CAD build for the part. Positions are in the model's coordinates, mm. A direction names the side the tool comes from. Coordinates: 2 decimals unless noted, no trailing zeros. Order: outer loops, then holes, each group sorted by start corner. A loop starts at its lowest first (then second) coordinate and runs counter-clockwise, first axis right, second up. Notation, with made-up numbers: M 24,58 L 82,58 A22 ccw 82,96 Z; hole C -5.5,59 d8. An arc over 180 degrees is marked long. One line per item, written item: value.
from build123d import *

# Parameters (mm, degrees)
F0_W     = 87.5153616071
F0_H     = 111.0227331519
F1_DEPTH = 60.452
F2_W     = 61.5649223328
F2_H     = 93.4719592333
F3_DEPTH = 25.4
F4_DEPTH = 25.4
F5_DEPTH = 25.4
F6_R     = 10.9826729048
F7_DEPTH = 111.0237331519
F8_W     = 35.9690990299
F8_H     = 23.0667970557
F9_DEPTH = 87.5163616071


with BuildPart() as f1:
    # F0 (on Top) → F1 (new body)
    with BuildSketch(Plane.XY):
        Rectangle(F0_W, F0_H)
    extrude(amount=F1_DEPTH)

    # F2 (on face) → F3 (cut)
    with BuildSketch(Plane.XY.offset(60.452)):
        Rectangle(F2_W, F2_H)
    extrude(amount=-F3_DEPTH, mode=Mode.SUBTRACT)

    # F4 (cut): a face of the model
    f4_faces = [f1.faces().sort_by_distance(p)[0] for p in [
        (0, 0, 35.052),
    ]]
    extrude(f4_faces, amount=-F4_DEPTH, mode=Mode.SUBTRACT)

    # F5 (cut): a face of the model
    f5_faces = [f1.faces().sort_by_distance(p)[0] for p in [
        (0, 0, 9.652),
    ]]
    extrude(f5_faces, amount=-F5_DEPTH, mode=Mode.SUBTRACT)

    # F6 (on face) → F7 (cut, through all)
    with BuildSketch(Plane(origin=(0, 55.511366576, 0), x_dir=(-1, 0, 0), z_dir=(0, 1, 0))):
        with Locations((0, 30.2436631173)):
            Circle(F6_R)
    extrude(amount=-F7_DEPTH, mode=Mode.SUBTRACT)

    # F8 (on face) → F9 (cut, through all)
    with BuildSketch(Plane(origin=(-43.7576808035, 0, 0), x_dir=(0, -1, 0), z_dir=(-1, 0, 0))):
        with Locations((0.5664424971, 48.9186014721)):
            Rectangle(F8_W, F8_H)
    extrude(amount=-F9_DEPTH, mode=Mode.SUBTRACT)


solid = f1.part
Q1. Which spindle directions (+Z, -Z, +X, -X, +Y, -Y) get a long thin tool onto all of the face, cutting with end or side? Do faces 1 (the face through (30.782, -1, 31)), 2 (the face through (37, 17.418, 49)), 3 (the face through (-10, 55.511, 37)). Say none if no direction does.
Recorded:
face 1: +Z, -Z
face 2: +Z, +X, -X
face 3: +Z, -Z, +X, -X, +Y
Q2. Mould opens along Y. For faces 4 (the face through (1.43, 51.185, 41.133)), 5 (the face through (-10, -55.511, 37)), 6 (the face through (-37, 0, 37.385)) say: released by +Y, released by -Y, zero draft, split by the parting line, or undercut.
Recorded:
face 4: zero draft
face 5: released by -Y
face 6: undercut
Q3. Slice it at B-B (y = -45). List the corners of the cut face in (x, z).
Recorded:
outline: M -43.76,0 L -30.78,0 L -30.78,60.45 L -43.76,60.45 Z; M 30.78,0 L 43.76,0 L 43.76,60.45 L 30.78,60.45 Z
Q4. Slice it at A-A (x = 0). List the corners of the cut face in (y, z), plus the area to 3 significant figures.
Recorded:
outline: M -55.51,0 L -46.74,0 L -46.74,19.26 L -55.51,19.26 Z; M -55.51,41.23 L -46.74,41.23 L -46.74,60.45 L -55.51,60.45 Z; M 46.74,0 L 55.51,0 L 55.51,19.26 L 46.74,19.26 Z; M 46.74,41.23 L 55.51,41.23 L 55.51,60.45 L 46.74,60.45 Z
area: 675 mm^2
Q5. Slice it at D-D (x = 25). List the corners of the cut face in (y, z), plus the area to 3 significant figures.
Recorded:
outline: M -55.51,0 L -46.74,0 L -46.74,60.45 L -55.51,60.45 Z; M 46.74,0 L 55.51,0 L 55.51,60.45 L 46.74,60.45 Z
area: 1,060 mm^2
Q6. Pin check, flat tips, straight feed: pin 1 Ø13 at (x, z) = (0, 30.24) entering from +Y; pin 2 Ø6.5 at (x, y) = (-39, -7.5) entering from +Z. Stop position of each tip, or through.
Recorded:
pin 1: passes through
pin 2: stops at z = 37.39
Q7. Drill centre lines: line 1 along Y through (x, z) = (18, 11); line 2 along Z through (x, y) = (0, -49.5); line 3 along X through (y, z) = (-21.5, 21). Where is each one in solid material? Low to high.
Recorded:
line 1: y = -55.51 to -46.74, 46.74 to 55.51
line 2: z = 0 to 19.26, 41.23 to 60.45
line 3: x = -43.76 to -30.78, 30.78 to 43.76
Q8. Slice it at C-C (z = 15.5). List the corners of the cut face in (x, y).
Recorded:
outline: M -43.76,-55.51 L 43.76,-55.51 L 43.76,55.51 L -43.76,55.51 Z; hole M -30.78,-46.74 L 30.78,-46.74 L 30.78,46.74 L -30.78,46.74 Z
